Part model, mm, in its own coordinate system. Round coordinates to 2 decimals unless told otherwise and drop trailing zeros. Write each loop counter-clockwise with the first axis right and the second up, starting at its lowest first coordinate (ties: lowest second). Pieces come first, ordered by that corner, then holes. Notation, with made-up numbers: M 67.25,73 L 124.25,73 A22 cw 124.25,80 Z; hole C 10,64.25 d3. An arc over 180 degrees is marked long. Use a Markdown table: item, result. Add a question column.
1) Slice it at B-B on x = -119. Write the cut outline in (y, z), plus the area to 3 significant figures.
2) Wall check: probe 1 along Y at (x, z) = (-8.5, -36); probe 2 along Z at (x, y) = (-117.5, -10.5); probe 3 along Z at (x, y) = (-8, -20.5). Give the ranges that are in metal, low to high.
3) Slice it at D-D on y = -134.5. Write the cut outline in (x, z), plus the area to 3 significant figures.
4) Slice it at C-C on z = -14.5. Write the cut outline in (x, y), plus the area to 3 significant figures.
5) Drop flat-ended pins along their axis: P1, Ø6, axis at x = -135, y = -56, coming from the -Z side; P2, Ø1, axis at x = -52, y = -98, coming from the -Z side; P3, Ø12, axis at x = -85, y = -88.5, coming from the -Z side. Give the stop position or say it passes through.
6) Two-plate mould, pull along Y, no slides. Class faces 1 (the face through (-57, -157, 13)), 2 (the face through (-56.53, -1.48, 111.88)), 3 (the face through (-59, -3, 13)), 4 (the face through (-60, 0, 12)): released by +Y, released by -Y, zero draft, split by the parting line, or undercut.
7) Slice it at A-A on z = 81.5. Write the cut outline in (x, y).
```python
from build123d import *

# Parameters (mm, degrees)
F1_DEPTH = 160
F4_DEPTH = 184


with BuildPart() as f1:
    # F0 (on Front) → F1 (new body)
    with BuildSketch(Plane.XZ):
        with BuildLine():
            Line((40.9332527794, -52.7619718481), (-48.0891487754, 106.7585873007))
            ThreePointArc((-48.0891487754, 106.7585873007), (-56.6755499732, 111.8843764566), (-65.4078141956, 107.0112294702))
            Line((-65.4078141956, 107.0112294702), (-159.0454700669, -49.8447113565))
            Line((-159.0454700669, -49.8447113565), (40.9332527794, -52.7619718481))
        make_face()
    extrude(amount=F1_DEPTH)

    # F3 (on offset) → F4 (cut)
    with BuildSketch(Plane(origin=(-0.7170523297, 0, -49.1540640703), x_dir=(0.9998936142, 0, -0.0145863025), z_dir=(-0.0145863025, 0, -0.9998936142))):
        Polygon((-161.2010151148, 3), (-155.3014998566, 3), (38.6985001434, 3), (52.8733432293, 3), (52.8733432293, 157), (38.6985001434, 157), (-155.3014998566, 157), (-161.2010151148, 157), align=None)
    extrude(amount=-F4_DEPTH, mode=Mode.SUBTRACT)


solid = f1.part
```
Entries:
| question | item | result |
|---|---|---|
| 1 | outline | M -160,-50.43 L 0,-50.43 L 0,17.24 L -3,17.24 L -3,-47.43 L -157,-47.43 L -157,17.24 L -160,17.24 Z |
| 1 | area | 868 mm^2 |
| 2 | probe 1 | y = -160 to -157, -3 to 0 |
| 2 | probe 2 | z = -50.45 to -47.45 |
| 2 | probe 3 | z = -52.05 to -49.05 |
| 3 | outline | M -159.05,-49.84 L 40.93,-52.76 L 39.25,-49.74 L -157.27,-46.87 Z |
| 3 | area | 595 mm^2 |
| 4 | outline | M -137.95,-160 L 19.58,-160 L 19.58,-157 L -137.95,-157 Z; M -137.95,-3 L 19.58,-3 L 19.58,0 L -137.95,0 Z |
| 4 | area | 945 mm^2 |
| 5 | P1 | stops at z = -50.24 |
| 5 | P2 | stops at z = -51.41 |
| 5 | P3 | stops at z = -51.01 |
| 6 | face 1 | undercut |
| 6 | face 2 | zero draft |
| 6 | face 3 | undercut |
| 6 | face 4 | released by +Y |
| 7 | outline | M -80.64,-160 L -33.99,-160 L -33.99,-157 L -80.64,-157 Z; M -80.64,-3 L -33.99,-3 L -33.99,0 L -80.64,0 Z |
